Here's the drawing with two shaded views (mm, measured from the low corner). I have some questions. A direction names the side the tool comes from. Round coordinates to 2 decimals unless told otherwise and drop trailing zeros. Loops run counter-clockwise (first coordinate to the right, second up) from the corner with the lowest first, then second, coordinate; pieces in that order, holes last. Notation, with made-up numbers: (-11.5, -34.5) - (38.5, -34.5) arc R17 cw to (38.5, -21.5) - close; hole circle Ø10 at (84, 33). An arc over 180 degrees is marked (long way). Answer as CSV lines item,"result".
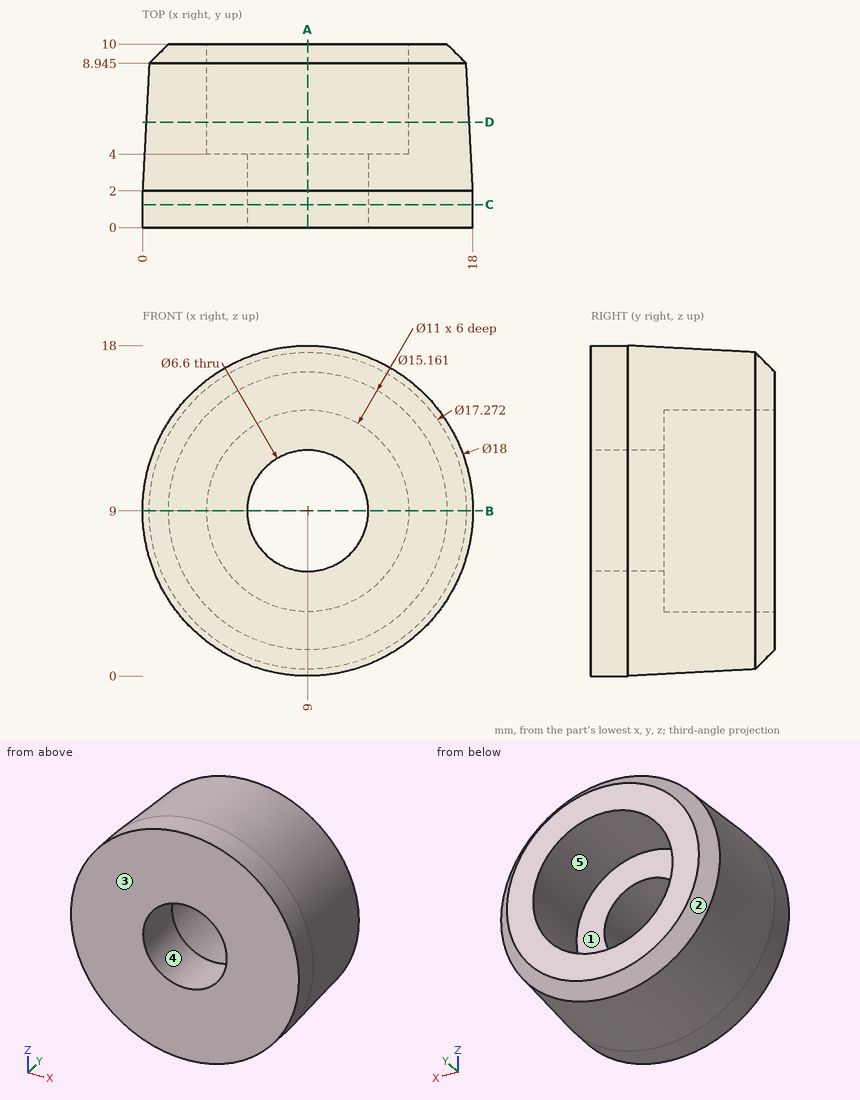
Q1. Imagine slicing it at D-D (y = 5.75). Write out the boundary of the cut face in (x, z).
Checks:
outline,"circle Ø17.61 at (9, 9); hole circle Ø11 at (9, 9)"
Q2. Imagine slicing it at C-C (y = 1.25). Write out the boundary of the cut face in (x, z), then the cut area to 3 significant figures.
Checks:
outline,"circle Ø18 at (9, 9); hole circle Ø6.6 at (9, 9)"
area,"220 mm²"
Q3. We'd pull the mould along Z, two halves only. Please class the marked faces 1, 2 and 3: pulls with the +Z half, pulls with the -Z half, needs draft (parallel to the pull), parting line crosses it, or undercut.
Checks:
face 1,"undercut"
face 2,"parting line crosses it"
face 3,"needs draft"
Q4. I'm going to push flat-ended pins straight in: pin 1 Ø6 at (y, z) = (8, 15.5) entering from -X; pin 2 Ø2 at (x, y) = (10, 4.5) entering from -Z; pin 3 Ø7.5 at (x, z) = (9, 9) entering from +Y. Where does each tip first touch, or does it pass through?
Checks:
pin 1,"x = 1.04"
pin 2,"z = 0.1"
pin 3,"y = 4"
Q5. Imagine slicing it at B-B (z = 9). Write out the boundary of the cut face in (x, y) (1 decimal).
Checks:
outline,"(0, 0) - (5.7, 0) - (5.7, 4) - (3.5, 4) - (3.5, 10) - (1.4, 10) - (0.4, 8.9) - (0, 2) - close; (12.3, 0) - (18, 0) - (18, 2) - (17.6, 8.9) - (16.6, 10) - (14.5, 10) - (14.5, 4) - (12.3, 4) - close"
Q6. On a 3-axis mill with a long thin cutter (end or side, diameter ignored), from which of +Z, -Z, +X, -X, +Y, -Y can I reach the whole of each face in a straight line? I mean the marked faces 4 and 5. Say none if no direction works.
Checks:
face 4,"+Y, -Y"
face 5,"+Y"
Q7. Imagine slicing it at A-A (x = 9). Write out the boundary of the cut face in (y, z) (1 decimal).
Checks:
outline,"(0, 0) - (2, 0) - (8.9, 0.4) - (10, 1.4) - (10, 3.5) - (4, 3.5) - (4, 5.7) - (0, 5.7) - close; (0, 12.3) - (4, 12.3) - (4, 14.5) - (10, 14.5) - (10, 16.6) - (8.9, 17.6) - (2, 18) - (0, 18) - close"
Q8. If I drill on line 1 along X through (y, z) = (0.9, 9); line 2 along Z through (x, y) = (9, 5.5), over which ranges is the centre line in solid material (lowest first)? Write a range as [from, to].
Checks:
line 1,"[0, 5.7], [12.3, 18]"
line 2,"[0.18, 3.5], [14.5, 17.82]"
